For this review, take the finished solid that the model builds, in its own axes (mm). A direction names the side the tool comes from. Coordinates: 2 decimals unless noted, no trailing zeros. Write each loop counter-clockwise with the first axis right and the second up, starting at its lowest first coordinate (ties: lowest second). Pieces come first, ordered by that corner, then holes. Notation, with made-up numbers: M 5.25,84.5 L 54.25,84.5 A27 ccw 54.25,111.5 Z; hole C 82,71 d8. An arc over 180 degrees is marked long. One line per question, with ' | ' between items.
Autodesk Inventor part; units mm, degrees
ref_plane "YZ Plane" through (0, 0, 0) normal (1, 0, 0) x (0, 1, 0)
ref_plane "XZ Plane" through (0, 0, 0) normal (0, 1, 0) x (-1, 0, 0)
ref_plane "XY Plane" through (0, 0, 0) normal (0, 0, 1) x (1, 0, 0)
sketch "Sketch1" plane through (0, 0, 0) normal (0, 1, 0) x (-1, 0, 0)
  circle A0 centre (0, 0) radius 51.5
  line L0 (-6.4, 6.4) -> (6.4, 6.4)
  line L1 (6.4, 6.4) -> (6.4, -6.4)
  line L2 (6.4, -6.4) -> (-6.4, -6.4)
  line L3 (-6.4, -6.4) -> (-6.4, 6.4)
  line L4 (-6.4, 6.4) -> (6.4, -6.4) construction
  line L5 (6.4, 6.4) -> (-6.4, -6.4) construction
  dimension "d0" = 103
  dimension "d1" = 12.8
  dimension "d2" = 12.8
extrude "Extrusion1" add sketch "Sketch1" along normal blind 3
sketch "Sketch2" plane through (0, 3, 0) normal (0, 1, 0) x (1, 0, 0)
  line L0 (-6.4, -6.4) -> (-6.4, 6.4) construction
  line L1 (-6.4, 6.4) -> (6.4, 6.4) construction
  line L2 (6.4, 6.4) -> (6.4, -6.4) construction
  line L3 (6.4, -6.4) -> (-6.4, -6.4) construction
  circle A0 centre (0, 0) radius 51.5 construction
  line L4 (6.4, 0) -> (51.5, 0) construction
  circle A1 centre (0, 0) radius 51.5 construction
  line L5 (0, 0) -> (-25.75, 44.6003) construction
  line L6 (0, 0) -> (-25.75, -44.6003) construction
  circle A2 centre (0, 0) radius 45 construction
  line L7 (0, 0) -> (0, -51.5) construction
  line L8 (0, 0) -> (44.6003, -25.75) construction
  line L9 (0, 0) -> (25.75, -44.6003) construction
  line L10 (0, 0) -> (25.75, 44.6003) construction
  line L11 (44.6003, 25.75) -> (0, 0) construction
  line L12 (0, 0) -> (0, 51.5) construction
  line L13 (0, 0) -> (-44.6003, -25.75) construction
  line L14 (0, 0) -> (-51.5, 0) construction
  line L15 (0, 0) -> (-44.6003, 25.75) construction
  circle A3 centre (38.9711, -22.5) radius 1.5
  circle A4 centre (22.5, -38.9711) radius 1.5
  circle A5 centre (0, -45) radius 1.5
  circle A6 centre (-38.9711, -22.5) radius 1.5
  circle A7 centre (-45, 0) radius 1.5
  circle A8 centre (-38.9711, 22.5) radius 1.5
  circle A9 centre (22.5, 38.9711) radius 1.5
  circle A10 centre (38.9711, 22.5) radius 1.5
  circle A11 centre (0, 45) radius 1.5
  dimension "d7" = 90
  dimension "d5" = 120
  dimension "d6" = 120
  dimension "d8" = 30
  dimension "d9" = 30
  dimension "d10" = 30
  dimension "d11" = 30
  dimension "d12" = 30
  dimension "d13" = 30
  dimension "d14" = 30
  dimension "d15" = 30
  dimension "d16" = 3
  dimension "d17" = 3
  dimension "d18" = 3
  dimension "d19" = 3
  dimension "d20" = 3
  dimension "d21" = 3
  dimension "d22" = 3
  dimension "d23" = 3
  dimension "d24" = 3
extrude "Extrusion2" cut sketch "Sketch2" against normal blind 3
sketch "Sketch3" plane through (0, 0, 0) normal (0, -1, 0) x (1, 0, 0)
  circle A0 centre (38.9711, -22.5) radius 1.5
  circle A1 centre (-38.9711, -22.5) radius 1.5
  circle A2 centre (-38.9711, 22.5) radius 1.5
  circle A3 centre (22.5, 38.9711) radius 1.5
  circle A4 centre (38.9711, 22.5) radius 1.5
  circle A5 centre (0, 45) radius 1.5
  circle A6 centre (-45, 0) radius 1.5
  circle A7 centre (22.5, -38.9711) radius 1.5
  circle A8 centre (0, -45) radius 1.5
  line L0 (-6.4, -6.4) -> (-6.4, 6.4)
  line L1 (-6.4, 6.4) -> (6.4, 6.4)
  line L2 (6.4, 6.4) -> (6.4, -6.4)
  line L3 (6.4, -6.4) -> (-6.4, -6.4)
  circle A9 centre (0, 0) radius 51.5
equation "\"d2\" = d1"
equation "\"d9\" = d8"
equation "\"d10\" = d8"
equation "\"d11\" = d8"
equation "\"d12\" = d8"
equation "\"d13\" = d8"
equation "\"d14\" = d8"
equation "\"d15\" = d8"
equation "\"d17\" = d16"
equation "\"d18\" = d16"
equation "\"d19\" = d16"
equation "\"d20\" = d16"
equation "\"d21\" = d16"
equation "\"d22\" = d16"
equation "\"d23\" = d16"
equation "\"d24\" = d16"
properties part number "top top plate" material "Polycarbonate, Clear"
1) To check wall thickness, follow line 1 along Z through (x, y) = (0, 2.2); line 2 along Z through (x, y) = (22.5, 2); line 3 along Z through (x, y) = (22, 2.65). State the ranges of each line that lie inside material, in increasing order. Write a range as [from, to].
Responses:
line 1: [-51.5, -46.5], [-43.5, -6.4], [6.4, 43.5], [46.5, 51.5] | line 2: [-46.32, -40.47], [-37.47, 37.47], [40.47, 46.32] | line 3: [-46.56, -40.39], [-37.56, 37.56], [40.39, 46.56]
2) Machinability: for faces 1 (the flat face through (1, 0, -11)), 2 (the flat face through (-6.4, 1, 0)), which of the approach directions +Z, -Z, +X, -X, +Y, -Y give a long, thin tool a straight path to every point of the face, cutting with its end or side? Answer none if there is none.
Responses:
face 1: +Z, -Z, +X, -X, -Y | face 2: +Y, -Y
3) Insertion check: pin 1 Ø3.5 at (x, z) = (0, -45) entering from +Y; pin 2 Ø0.9 at (x, y) = (3, 1) entering from +Z; pin 3 Ø1.5 at (x, y) = (2.5, 1) entering from -Z. Each pin has a flat end and moves straight along its axis. Give the tip position at first contact, or say it passes through.
Responses:
pin 1: y = 3 | pin 2: z = 51.44 | pin 3: z = -51.47
4) The part is to be moulded in two halves that separate along Z. For faces 3 (the flat face through (6.4, 1, 0)), 4 (the cylindrical face through (11.164, 1.479, 50.275)), 5 (the flat face through (1, 3, -11)), say which applies: +Z half, -Z half, draft (parallel to the pull), parting line (faces both ways), or undercut.
Responses:
face 3: undercut | face 4: parting line | face 5: draft
5) We need section D-D on y = 1.2. State how many separate pieces and enclosed holes the cut face has, then the cut area to 3 significant figures.
Responses:
separate pieces: 1 | enclosed holes: 10 | area: 8,100 mm^2
6) We need section C-C on x = 22.5. State the section outline as (y, z) points.
Responses:
outline: M 0,-46.32 L 3,-46.32 L 3,-40.47 L 0,-40.47 Z; M 0,-37.47 L 3,-37.47 L 3,37.47 L 0,37.47 Z; M 0,40.47 L 3,40.47 L 3,46.32 L 0,46.32 Z
7) We need section A-A on x = 0. State the section outline as (y, z) points, then the cut area to 3 significant figures.
Responses:
outline: M 0,-51.5 L 3,-51.5 L 3,-46.5 L 0,-46.5 Z; M 0,-43.5 L 3,-43.5 L 3,-6.4 L 0,-6.4 Z; M 0,6.4 L 3,6.4 L 3,43.5 L 0,43.5 Z; M 0,46.5 L 3,46.5 L 3,51.5 L 0,51.5 Z | area: 253 mm^2
8) We need section B-B on z = 0. State the section outline as (x, y) points.
Responses:
outline: M -51.5,0 L -46.5,0 L -46.5,3 L -51.5,3 Z; M -43.5,0 L -6.4,0 L -6.4,3 L -43.5,3 Z; M 6.4,0 L 51.5,0 L 51.5,3 L 6.4,3 Z
